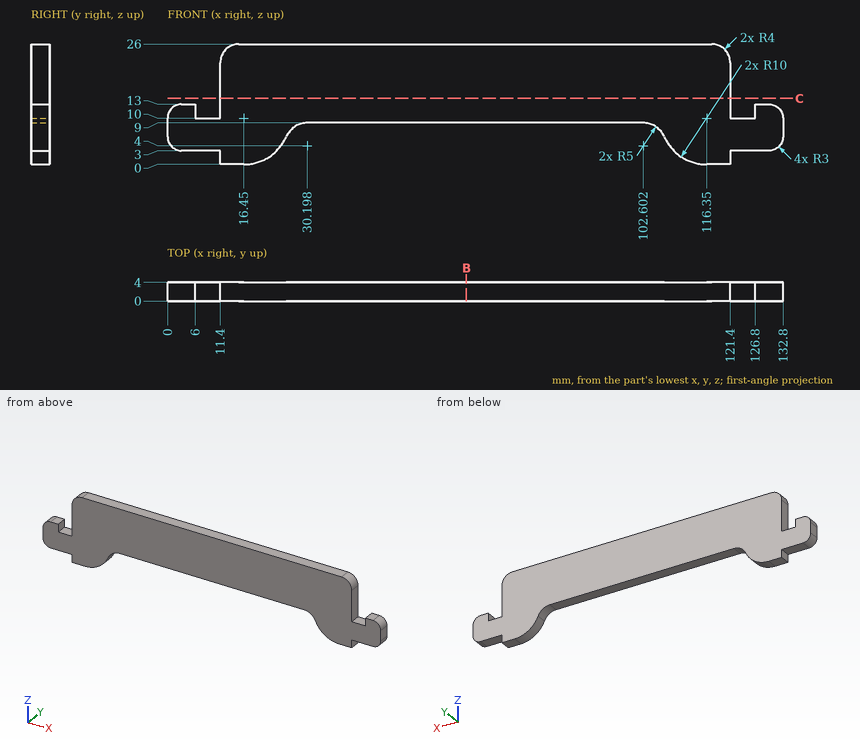
Study the drawing (mm; zero at the part's minimum x, y, z) and answer. Give positions to 0.01 mm unless a question says otherwise; leave off trailing zeros. Order: outer loops, then holes, each group sorted by start corner. A loop starts at its lowest first (then second) coordinate and runs counter-clockwise, first axis right, second up. Notation, with made-up numbers: (-31, 35.25) - (18, 35.25) arc R15 ccw to (18, 57.25) - close; hole circle Ø9 at (-23, 24.25). An arc over 180 degrees is marked (long way). Answer as CSV lines item,"result". Start each with the question number.
Q1. The part is cut by section B-B (x = 64.5). Write down the section's boundary in (y, z).
Q2. Given pin 1 Ø1 at (x, y) = (100, 0.5) entering from -Z; pin 2 Ø1.5 at (y, z) = (3, 12) entering from +X; pin 3 Ø1.5 at (y, z) = (1.5, 21.5) entering from +X, each flat-ended and moving along its own axis, determine where each tip first touches the part or whether it passes through.
Q3. Find the intervals of material crossed by L1, parallel to Z at x = 70.5, y = 2.85; L2, parallel to X at y = 1.7, z = 6.25; L3, parallel to X at y = 1.05, z = 2, in increasing order. Write a range as [from, to].
Q4. The part is cut by section C-C (z = 14.25). Write down the section's boundary in (x, y), then the cut area to 3 significant figures.
Check result:
1,outline,"(0, 9) - (4, 9) - (4, 26) - (0, 26) - close"
2,pin 1,"stops at z = 9"
2,pin 2,"stops at x = 132.53"
2,pin 3,"stops at x = 121.4"
3,L1,"z = [9, 26]"
3,L2,"x = [0, 25.73], [107.07, 132.8]"
3,L3,"x = [11.4, 22.45], [110.35, 121.4]"
4,outline,"(11.4, 0) - (121.4, 0) - (121.4, 4) - (11.4, 4) - close"
4,area,"440 mm²"
